Here's the drawing with two shaded views (mm, measured from the low corner). I have some questions. A direction names the side the tool comes from. Round coordinates to 2 decimals unless told otherwise and drop trailing zeros. Order: outer loops, then holes, each group sorted by start corner. A loop starts at its lowest first (then second) coordinate and runs counter-clockwise, first axis right, second up.
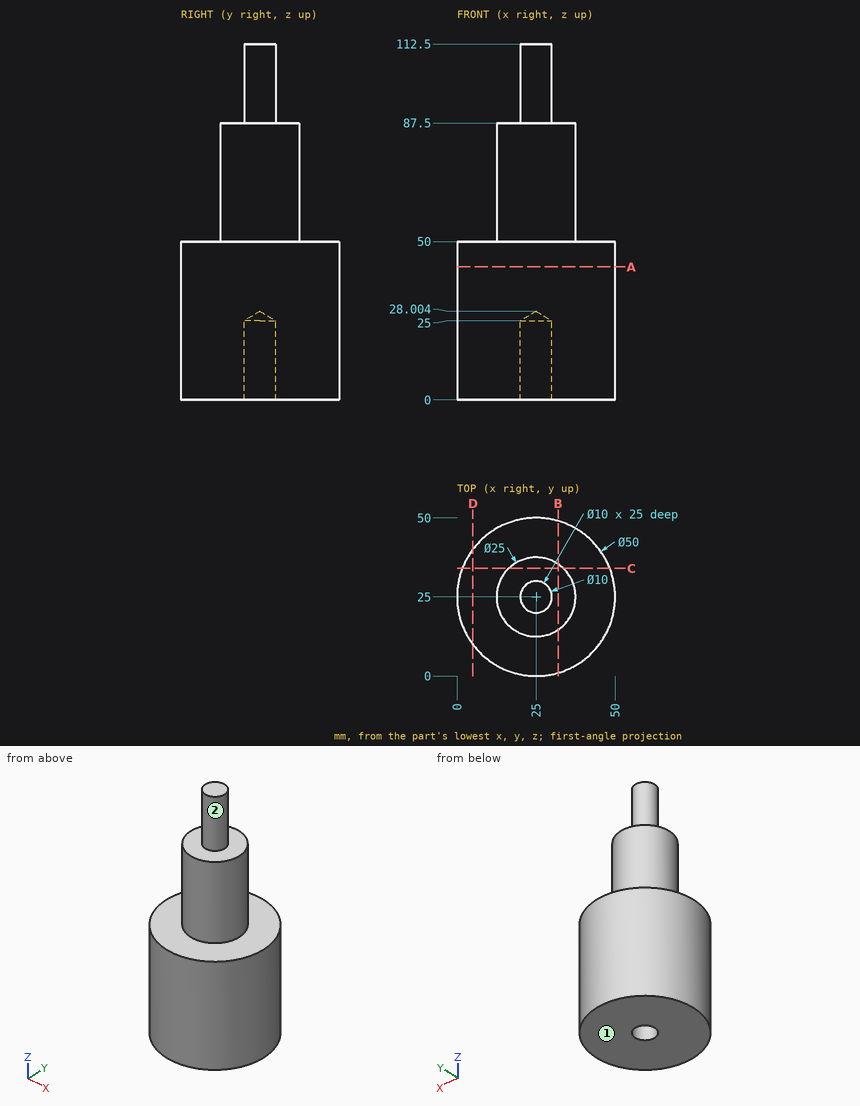
1. If we section it at A-A, the plane z = 42: Write out the boundary of the cut face in (x, y), and give its area (3 significant figures).
Evaluation:
outline: circle Ø50 at (25, 25)
area: 1,960 mm2
2. I'm going to push flat-ended pins straight in: P1, Ø2, axis at x = 32, z = 17.5, coming from the -Y side; P2, Ø12, axis at y = 32, z = 101, coming from the -X side; P3, Ø4, axis at x = 36, z = 58, coming from the -Y side (1 decimal); P4, Ø8, axis at y = 44.5, z = 70.5, coming from the +X side. Where does each tip first touch, or does it pass through?
Evaluation:
P1: stops at y = 0.73
P2: stops at x = 20.1
P3: stops at y = 16.3
P4: passes through
3. On a 3-axis mill with a long thin cutter (end or side, diameter ignored), from which of +Z, -Z, +X, -X, +Y, -Y can I reach the whole of each face in a straight line? I mean the marked faces 1 and 2. Say none if no direction works.
Evaluation:
face 1: -Z, +X, -X, +Y, -Y
face 2: +Z
4. If we section it at D-D, the plane x = 5: Write out the boundary of the cut face in (y, z).
Evaluation:
outline: (10, 0) - (40, 0) - (40, 50) - (10, 50) - close
5. If we section it at C-C, the plane y = 34: Write out the boundary of the cut face in (x, z) (1 decimal), and give its area (3 significant figures).
Evaluation:
outline: (1.7, 0) - (48.3, 0) - (48.3, 50) - (33.7, 50) - (33.7, 87.5) - (16.3, 87.5) - (16.3, 50) - (1.7, 50) - close
area: 2,980 mm2
6. If we section it at B-B, the plane x = 32: Write out the boundary of the cut face in (y, z), and give its area (3 significant figures).
Evaluation:
outline: (1, 0) - (49, 0) - (49, 50) - (35.36, 50) - (35.36, 87.5) - (14.64, 87.5) - (14.64, 50) - (1, 50) - close
area: 3,180 mm2
7. I need wall thicknesses on probe 1 along Y at (x, z) = (25, 8); probe 2 along Z at (x, y) = (44, 30.5); probe 3 along Z at (x, y) = (23.5, 15.5). Which ranges of each line are inside material? Lowest first, please.
Evaluation:
probe 1: y = 0 to 20, 30 to 50
probe 2: z = 0 to 50
probe 3: z = 0 to 87.5
